from build123d import *

# Parameters (mm, degrees)
F1_DEPTH      = 35
F2_W          = 25
F2_H          = 26
F3_DEPTH      = 10.001
F3_DEPTH_BACK = 10.201
F4_W          = 15
F4_H          = 6
F4_H_2        = 2.5
F5_DEPTH      = 6
F6_R          = 10
F7_DEPTH      = 4


with BuildPart() as f1:
    # F0 (on Right) → F1 (new body)
    with BuildSketch(Plane.YZ):
        Polygon((1.6723675691, 40), (-2.3276324309, 40), (-2.3276324309, 6), (-2.3276324309, 0), (11.8723675691, 0), (11.8723675691, 40), (7.8723675691, 40), (7.8723675691, 4), (1.6723675691, 4), align=None)
        Polygon((-2.3276324309, 0), (-2.3276324309, 6), (-4.3276324309, 6), (-4.3276324309, 8.5), (-5.8276324309, 8.5), (-8.3276324309, 6), (-8.3276324309, 0), align=None)
    extrude(amount=F1_DEPTH)

    # F2 (on face) → F3 (cut, two sides)
    with BuildSketch(Plane(origin=(0, 1.6723675691, 0), x_dir=(-1, 0, 0), z_dir=(0, 1, 0))) as f3_sk:
        with Locations((-17.5, 27)):
            Rectangle(F2_W, F2_H)
    extrude(amount=-F3_DEPTH, mode=Mode.SUBTRACT)
    extrude(f3_sk.sketch, amount=F3_DEPTH_BACK, mode=Mode.SUBTRACT)

    # F4 (on face) → F5 (cut, through all)
    with BuildSketch(Plane.XZ.offset(8.3276324309)):
        with Locations((17.5, 3)):
            Rectangle(F4_W, F4_H)
        with Locations((17.5, 7.25)):
            Rectangle(F4_W, F4_H_2)
    extrude(amount=-F5_DEPTH, mode=Mode.SUBTRACT)

    # F6 (on face) → F7 (cut, through all)
    with BuildSketch(Plane(origin=(0, 11.8723675691, 0), x_dir=(-1, 0, 0), z_dir=(0, 1, 0))):
        with Locations((-17.5, 14)):
            Circle(F6_R)
    extrude(amount=-F7_DEPTH, mode=Mode.SUBTRACT)


solid = f1.part
For this review, take the finished solid that the model builds, in its own axes (mm). A direction names the side the tool comes from. Give positions to 0.01 mm unless a question says otherwise; leave off trailing zeros. Write each loop counter-clockwise with the first axis right and the second up, starting at its lowest first coordinate (ties: lowest second). Pieces come first, ordered by that corner, then holes. Notation, with made-up numbers: (40, -3) -> (55, -3) arc R17 ccw to (55, 23) -> close; hole circle Ø1 at (43.25, -29.75). An arc over 180 degrees is marked (long way). Use CSV: the item, a comma, the result in double quotes.
Q1. Take a section at A-A, the plane z = 15.5. Write out the cut boundary in (x, y).
Conclusion:
outline,"(0, -2.33) -> (5, -2.33) -> (5, 1.67) -> (0, 1.67) -> close; (0, 7.87) -> (5, 7.87) -> (5, 11.87) -> (0, 11.87) -> close; (30, -2.33) -> (35, -2.33) -> (35, 1.67) -> (30, 1.67) -> close; (30, 7.87) -> (35, 7.87) -> (35, 11.87) -> (30, 11.87) -> close"
Q2. Tool access review of faces 1 (the face through (17.7, 9.9, 4)), 2 (the face through (5, 0, 27)), 3 (the face through (10, -5, 3)), 4 (the face through (17.3, 1.672, 13.7)): name each direction out of +Z, -Z, +X, -X, +Y, -Y from which nothing blocks a thin tool from reaching the whole face with its end or side.
Conclusion:
face 1,"+Z, +Y"
face 2,"+Z, +Y, -Y"
face 3,"+Z, -Z, -Y"
face 4,"+Z, +X, -X"
Q3. Mouldability with a two-part tool opening along Y and no side actions: class faces 5 (the face through (2, 0, 40)), 6 (the face through (30, -4.328, 7)), 7 (the face through (3, 7.872, 22)), 8 (the face through (5, -8.328, 3)) as pulls with the +Y half, pulls with the -Y half, needs draft (parallel to the pull), parting line crosses it, or undercut.
Conclusion:
face 5,"needs draft"
face 6,"undercut"
face 7,"undercut"
face 8,"pulls with the -Y half"
Q4. Take a section at D-D, the plane z = 5.5. Write out the cut boundary in (x, y), then the cut area to 3 significant figures.
Conclusion:
outline,"(0, -8.33) -> (10, -8.33) -> (10, -2.33) -> (25, -2.33) -> (25, -8.33) -> (35, -8.33) -> (35, 1.67) -> (0, 1.67) -> close; (0, 7.87) -> (12.23, 7.87) -> (12.23, 11.87) -> (0, 11.87) -> close; (22.77, 7.87) -> (35, 7.87) -> (35, 11.87) -> (22.77, 11.87) -> close"
area,"358 mm2"
Q5. To check wall thickness, follow probe 1 along X at (y, z) = (8.5, 17.5); probe 2 along Y at (x, z) = (2, 32.5); probe 3 along Z at (x, y) = (16, 3). State the ranges of each line that lie inside material, in increasing order. Write a range as [from, to].
Conclusion:
probe 1,"[0, 5], [30, 35]"
probe 2,"[-2.33, 1.67], [7.87, 11.87]"
probe 3,"[0, 4]"
Q6. Take a section at C-C, the plane y = -1.5. Write out the cut boundary in (x, z).
Conclusion:
outline,"(0, 0) -> (35, 0) -> (35, 40) -> (30, 40) -> (30, 14) -> (5, 14) -> (5, 40) -> (0, 40) -> close"
Q7. Take a section at B-B, the plane x = 9.5. Write out the cut boundary in (y, z).
Conclusion:
outline,"(-8.33, 0) -> (11.87, 0) -> (11.87, 8) -> (7.87, 8) -> (7.87, 4) -> (1.67, 4) -> (1.67, 14) -> (-2.33, 14) -> (-2.33, 6) -> (-4.33, 6) -> (-4.33, 8.5) -> (-5.83, 8.5) -> (-8.33, 6) -> close"
Q8. For P1, Ø14, axis at x = 30.5, z = 31, coming from the -Y side; P2, Ø1.2, axis at x = 6, y = 10, coming from the +Z side; P3, Ø1, axis at y = 2.5, z = 34, coming from the -X side; P4, Ø1, axis at x = 23.5, y = 5.5, coming from the +Z side, all flat-tipped, find the tip position at first contact; note any pin that passes through.
Conclusion:
P1,"y = -2.33"
P2,"z = 14"
P3,"through"
P4,"z = 4"
